Can you work these out from the model? Positions are in its coordinate system, mm. Face numbers are marked on the shaded views. A direction names the side the tool comes from. Give positions to 0.01 mm unless a question says otherwise; leave off trailing zeros. Loops run counter-clockwise (first coordinate to the right, second up) from the corner with the lowest first, then second, coordinate; pieces in that order, holes last. Notation, with made-up numbers: (-26, 36.25) - (-2, 36.25) arc R22 ccw to (-2, 69.25) - close; hole circle Ø7 at (26.25, -19.75). An arc over 180 degrees is marked (long way). Answer in a Markdown table with one row per item.
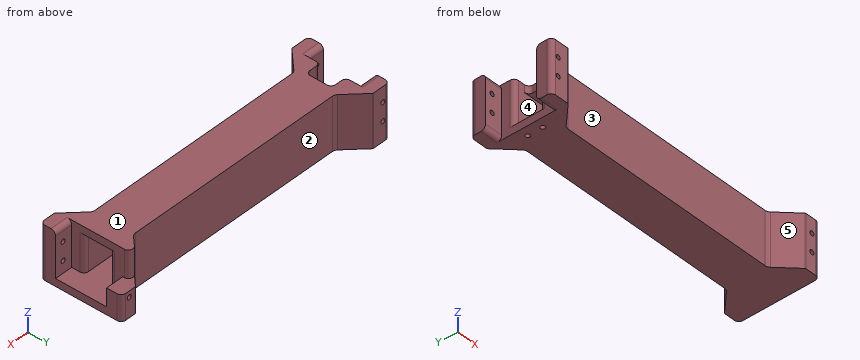
from build123d import *

# Parameters (mm, degrees)
EXTRUDE_1_DEPTH          = 35
SKETCH_2_W               = 25
SKETCH_2_H               = 17
CUT_EXTRUDE_1_DEPTH      = 211.274969583
SKETCH_3_W               = 25
SKETCH_3_H               = 8.5
CUT_EXTRUDE_2_DEPTH      = 12
FILLET_1_R               = 3
CUT_EXTRUDE_3_DEPTH      = 246.07389189
CUT_EXTRUDE_3_DEPTH_BACK = 246.07389189
SKETCH_4_R               = 1.5
CUT_EXTRUDE_4_DEPTH      = 10
FILLET_2_R               = 3
SKETCH_7_W               = 12
SKETCH_7_H               = 3
CUT_EXTRUDE_6_DEPTH      = 18
FILLET_3_R               = 3
CUT_EXTRUDE_8_DEPTH      = 10
FILLET_4_R               = 3
SKETCH_9_R               = 1.5
CUT_EXTRUDE_9_DEPTH      = 8
CUT_EXTRUDE_10_DEPTH     = 8
FILLET_5_R               = 3


with BuildPart() as part:
    # 草图1 → 凸台-拉伸1 (new body)
    with BuildSketch(Plane.XY):
        with BuildLine():
            Line((49.121689234, 57), (37.121689234, 57))
            Line((37.121689234, 57), (37.121689234, 3))
            Line((37.121689234, 3), (49.121689234, 3))
            ThreePointArc((49.121689234, 3), (49.40357385, 3.056070336), (49.642544089, 3.215745145))
            Line((49.642544089, 3.215745145), (61.832374142, 15.405575199))
            ThreePointArc((61.832374142, 15.405575199), (63.044614428, 16.215568261), (64.474549341, 16.5))
            Line((64.474549341, 16.5), (211.121689234, 16.5))
            ThreePointArc((211.121689234, 16.5), (212.551624147, 16.215568261), (213.763864432, 15.405575199))
            Line((213.763864432, 15.405575199), (225.953694486, 3.215745145))
            ThreePointArc((225.953694486, 3.215745145), (226.192664725, 3.056070336), (226.474549341, 3))
            Line((226.474549341, 3), (236.474549341, 3))
            Line((236.474549341, 3), (236.474549341, 57))
            Line((236.474549341, 57), (226.474549341, 57))
            ThreePointArc((226.474549341, 57), (226.192664725, 56.943929664), (225.953694486, 56.784254855))
            Line((225.953694486, 56.784254855), (213.763864432, 44.594424801))
            ThreePointArc((213.763864432, 44.594424801), (212.551624147, 43.784431739), (211.121689234, 43.5))
            Line((211.121689234, 43.5), (64.474549341, 43.5))
            ThreePointArc((64.474549341, 43.5), (63.044614428, 43.784431739), (61.832374142, 44.594424801))
            Line((61.832374142, 44.594424801), (49.642544089, 56.784254855))
            ThreePointArc((49.642544089, 56.784254855), (49.40357385, 56.943929664), (49.121689234, 57))
        make_face()
    extrude(amount=-EXTRUDE_1_DEPTH)

    # 草图2 → 切除-拉伸1 (cut, through all)
    with BuildSketch(Plane.ZY.offset(-37.121689234)):
        with Locations((-17.5, 30)):
            Rectangle(SKETCH_2_W, SKETCH_2_H)
    extrude(amount=-CUT_EXTRUDE_1_DEPTH, mode=Mode.SUBTRACT)

    # 草图3 → 切除-拉伸2 (cut)
    with BuildSketch(Plane.ZY.offset(-37.121689234)):
        with Locations((-17.5, 42.75)):
            Rectangle(SKETCH_3_W, SKETCH_3_H)
        with Locations((-17.5, 17.25)):
            Rectangle(SKETCH_3_W, SKETCH_3_H)
    cut_extrude_2 = extrude(amount=-CUT_EXTRUDE_2_DEPTH, mode=Mode.SUBTRACT)

    # 镜向1: 切除-拉伸2 across plane
    add(cut_extrude_2.mirror(Plane.ZY.offset(-136.798119287)), mode=Mode.SUBTRACT)

    # 圆角1
    fillet_1_edges = [part.edges().sort_by_distance(p)[0] for p in [
        (224.474549341, 38.5, -17.5),
        (224.474549341, 21.5, -17.5),
        (37.121689234, 3, -17.5),
        (37.121689234, 57, -17.5),
        (236.474549341, 57, -17.5),
        (236.474549341, 3, -17.5),
        (49.121689234, 38.5, -17.5),
        (49.121689234, 21.5, -17.5),
    ]]
    fillet(fillet_1_edges, radius=FILLET_1_R)

    # 草图4 → 切除-拉伸3 (cut, two sides: drawn at the far end of the back side and taken through both)
    with BuildSketch(Plane(origin=(0, 57, 0), x_dir=(1, 0, 0), z_dir=(0, 1, 0)).offset(-CUT_EXTRUDE_3_DEPTH_BACK)):
        with Locations(Location((42, 22, 0), (0, 0, 180))):
            Circle(SKETCH_4_R)
        with Locations(Location((42, 10, 0), (0, 0, 180))):
            Circle(SKETCH_4_R)
        with Locations(Location((230.798119287, 22, 0), (0, 0, 180))):
            Circle(SKETCH_4_R)
        with Locations(Location((230.798119287, 10, 0), (0, 0, 180))):
            Circle(SKETCH_4_R)
    extrude(amount=CUT_EXTRUDE_3_DEPTH + CUT_EXTRUDE_3_DEPTH_BACK, mode=Mode.SUBTRACT)

    # 草图5 → 切除-拉伸4 (cut)
    with BuildSketch(Plane(origin=(0, 0, -5), x_dir=(-1, 0, 0), z_dir=(0, 0, -1))):
        Polygon((-224.474549341, 41.5), (-224.474549341, 18.5), (-224.474549341, 13), (-236.474549341, 13), (-236.474549341, 47), (-224.474549341, 47), align=None)
        Polygon((-49.121689234, 41.5), (-49.121689234, 18.5), (-49.121689234, 13), (-37.121689234, 13), (-37.121689234, 47), (-49.121689234, 47), align=None)
    extrude(amount=-CUT_EXTRUDE_4_DEPTH, mode=Mode.SUBTRACT)

    # 圆角2
    fillet_2_edges = [part.edges().sort_by_distance(p)[0] for p in [
        (230.474549341, 13, 0),
        (230.474549341, 47, 0),
        (43.121689234, 47, 0),
        (43.121689234, 13, 0),
    ]]
    fillet(fillet_2_edges, radius=FILLET_2_R)

    # 草图7 → 切除-拉伸6 (cut)
    with BuildSketch(Plane.XY):
        with Locations((230.474549341, 48.5)):
            Rectangle(SKETCH_7_W, SKETCH_7_H)
        with BuildLine():
            Line((224.474549341, 50), (236.474549341, 50))
            Line((236.474549341, 50), (236.474549341, 54))
            ThreePointArc((236.474549341, 54), (235.595869685, 56.121320344), (233.474549341, 57))
            Line((233.474549341, 57), (226.474549341, 57))
            ThreePointArc((226.474549341, 57), (226.192664725, 56.943929664), (225.953694486, 56.784254855))
            Line((225.953694486, 56.784254855), (224.474549341, 55.30510971))
            Line((224.474549341, 55.30510971), (224.474549341, 50))
        make_face()
    extrude(amount=-CUT_EXTRUDE_6_DEPTH, mode=Mode.SUBTRACT)

    # 圆角3
    fillet_3_edges = [part.edges().sort_by_distance(p)[0] for p in [
        (224.474549341, 55.30510971, -9),
    ]]
    fillet(fillet_3_edges, radius=FILLET_3_R)

    # 草图8 → 切除-拉伸8 (cut)
    with BuildSketch(Plane.XY.offset(-30)):
        Polygon((49.121689234, 41.5), (49.121689234, 18.5), (49.121689234, 13), (37.121689234, 13), (37.121689234, 47), (49.121689234, 47), align=None)
    extrude(amount=-CUT_EXTRUDE_8_DEPTH, mode=Mode.SUBTRACT)

    # 圆角4
    fillet_4_edges = [part.edges().sort_by_distance(p)[0] for p in [
        (43.121689234, 13, -35),
        (43.121689234, 47, -35),
    ]]
    fillet(fillet_4_edges, radius=FILLET_4_R)

    # 草图9 → 切除-拉伸9 (cut)
    with BuildSketch(Plane(origin=(0, 0, -35), x_dir=(-1, 0, 0), z_dir=(0, 0, -1))):
        with Locations((-55.191240802, 25)):
            Circle(SKETCH_9_R)
        with Locations((-55.191240802, 35)):
            Circle(SKETCH_9_R)
    extrude(amount=-CUT_EXTRUDE_9_DEPTH, mode=Mode.SUBTRACT)

    # 草图10 → 切除-拉伸10 (cut)
    with BuildSketch(Plane(origin=(0, 0, -5), x_dir=(-1, 0, 0), z_dir=(0, 0, -1))):
        with BuildLine():
            Line((-52.121689234, 38.5), (-59.586907824, 38.5))
            Line((-59.586907824, 38.5), (-59.586907824, 21.5))
            Line((-59.586907824, 21.5), (-52.121689234, 21.5))
            ThreePointArc((-52.121689234, 21.5), (-50.00036889, 20.621320344), (-49.121689234, 18.5))
            Line((-49.121689234, 18.5), (-49.121689234, 41.5))
            ThreePointArc((-49.121689234, 41.5), (-50.00036889, 39.378679656), (-52.121689234, 38.5))
        make_face()
    extrude(amount=-CUT_EXTRUDE_10_DEPTH, mode=Mode.SUBTRACT)

    # 圆角5
    fillet_5_edges = [part.edges().sort_by_distance(p)[0] for p in [
        (59.586907824, 38.5, -2.5),
        (59.586907824, 21.5, -2.5),
    ]]
    fillet(fillet_5_edges, radius=FILLET_5_R)


solid = part.part
Q1. Imagine slicing it at B-B, the plane x = 135. Write out the boundary of the cut face in (y, z).
Checked values:
| item | result |
|---|---|
| outline | (16.5, -35) - (43.5, -35) - (43.5, 0) - (16.5, 0) - close; hole (21.5, -30) - (38.5, -30) - (38.5, -5) - (21.5, -5) - close |
Q2. If I drill on line 1 (Z direction, x = 42, y = 9); line 2 (Y direction, x = 175.5, z = -19); line 3 (Z direction, x = 119.5, y = 25), over which ranges is the centre line in solid material (lowest first)? Write a range as [from, to].
Checked values:
| item | result |
|---|---|
| line 1 | z = [-35, -23.5], [-20.5, -11.5], [-8.5, 0] |
| line 2 | y = [16.5, 21.5], [38.5, 43.5] |
| line 3 | z = [-35, -30], [-5, 0] |
Q3. On a 3-axis mill with a long thin cutter (end or side, diameter ignored), from which of +Z, -Z, +X, -X, +Y, -Y can I reach the whole of each face in a straight line? I mean the marked faces 1, 2 and 3. Say none if no direction works.
Checked values:
| item | result |
|---|---|
| face 1 | +Z, +X, -X, +Y, -Y |
| face 2 | +Z, -Z, +Y |
| face 3 | +Z, -Z, -Y |
Q4. Imagine slicing it at A-A, the plane y = 29. Write out the boundary of the cut face in (x, z).
Checked values:
| item | result |
|---|---|
| outline | (49.12, -35) - (236.47, -35) - (236.47, -30) - (49.12, -30) - close; (59.59, -5) - (224.47, -5) - (224.47, 0) - (59.59, 0) - close |
Q5. If we mould it in two halves opening along X, with no side actions, what happens to the marked faces 4 and 5? For each: released by +X, released by -X, zero draft, split by the parting line, or undercut.
Checked values:
| item | result |
|---|---|
| face 4 | zero draft |
| face 5 | undercut |
Q6. For pin 1 (2.5 mm diameter, centred on x = 42, z = -10, fed in from +Y); pin 2 (1 mm diameter, centred on y = 48, z = -11.5, fed in from +X); pin 3 (5 mm diameter, centred on x = 215.5, z = -7.5, fed in from +Y); pin 4 (2 mm diameter, centred on x = 161.5, z = -17, fed in from -Y), each with a flat end and sliding along its axis, tell me the tip position at first contact or that it passes through.
Checked values:
| item | result |
|---|---|
| pin 1 | passes through |
| pin 2 | stops at x = 224.47 |
| pin 3 | stops at y = 48.83 |
| pin 4 | stops at y = 16.5 |
